```python
from build123d import *

# Parameters (mm, degrees)
F0_W           = 152.4
F0_H           = 134.62
F1_DEPTH       = 6.35
F3_D           = 3.9878
F3_CBORE_D     = 7.112
F3_CBORE_DEPTH = 4.000000001
F4_T1_DEPTH    = 124.46
F4_T3_DEPTH    = 142.24
F4_T5_DEPTH    = 13.97
F4_S9_W        = 5.08
F4_S9_H        = 5.08
F4_T10_DEPTH   = 5.08
F4_S15_W       = 5.08
F4_S15_H       = 5.08
F4_T16_DEPTH   = 5.08
F4_S21_W       = 5.08
F4_S21_H       = 5.08
F4_T22_DEPTH   = 5.08
F4_S27_W       = 5.08
F4_S27_H       = 5.08
F4_T28_DEPTH   = 5.08


# Not quite as in the source:
# - a fillet or chamfer that OpenCascade refuses, or shapes differently, is made with other operations: its cross-section is extruded or revolved along the edge and cut away or added
# - a feature names something its author has since deleted; it is built from what else it names


with BuildPart() as f1:
    # F0 (on Top) → F1 (new body)
    with BuildSketch(Plane.XY):
        Rectangle(F0_W, F0_H)
    extrude(amount=F1_DEPTH)

    # F3 (through all)
    with Locations(Plane.XY.offset(6.35)):
        with Locations((-72.39, 41.91), (-72.39, -34.29), (72.39, -34.29), (72.39, 41.91)):
            CounterBoreHole(F3_D / 2, F3_CBORE_D / 2, F3_CBORE_DEPTH)

    # F4: fillet of radius 5.08 on 8 edges, made by hand

    # F4_s2 → F4_t1 (cut)
    with BuildSketch(Plane.XZ.offset(-62.23)):
        with BuildLine():
            ThreePointArc((-76.2, 1.27), (-74.7121024484, 4.8621024484), (-71.12, 6.35))
            Line((-71.12, 6.35), (-76.2, 6.35))
            Line((-76.2, 6.35), (-76.2, 1.27))
        make_face()
        with BuildLine():
            ThreePointArc((76.2, 1.27), (74.7121024484, 4.8621024484), (71.12, 6.35))
            Line((71.12, 6.35), (76.2, 6.35))
            Line((76.2, 6.35), (76.2, 1.27))
        make_face()
    extrude(amount=F4_T1_DEPTH, mode=Mode.SUBTRACT)

    # F4_s4 → F4_t3 (cut)
    with BuildSketch(Plane.YZ.offset(-71.12)):
        with BuildLine():
            ThreePointArc((62.23, 6.35), (65.8221024484, 4.8621024484), (67.31, 1.27))
            Line((67.31, 1.27), (67.31, 6.35))
            Line((67.31, 6.35), (62.23, 6.35))
        make_face()
        with BuildLine():
            ThreePointArc((-67.31, 1.27), (-65.8221024484, 4.8621024484), (-62.23, 6.35))
            Line((-62.23, 6.35), (-67.31, 6.35))
            Line((-67.31, 6.35), (-67.31, 1.27))
        make_face()
    extrude(amount=F4_T3_DEPTH, mode=Mode.SUBTRACT)

    # F4_s6 → F4_t5 (cut)
    with BuildSketch(Plane.XY.offset(-12.7)):
        with BuildLine():
            ThreePointArc((-71.12, -67.31), (-74.7121024484, -65.8221024484), (-76.2, -62.23))
            Line((-76.2, -62.23), (-76.2, -67.31))
            Line((-76.2, -67.31), (-71.12, -67.31))
        make_face()
        with BuildLine():
            ThreePointArc((71.12, -67.31), (74.7121024484, -65.8221024484), (76.2, -62.23))
            Line((76.2, -62.23), (76.2, -67.31))
            Line((76.2, -67.31), (71.12, -67.31))
        make_face()
        with BuildLine():
            ThreePointArc((76.2, 62.23), (74.7121024484, 65.8221024484), (71.12, 67.31))
            Line((71.12, 67.31), (76.2, 67.31))
            Line((76.2, 67.31), (76.2, 62.23))
        make_face()
        with BuildLine():
            ThreePointArc((-76.2, 62.23), (-74.7121024484, 65.8221024484), (-71.12, 67.31))
            Line((-71.12, 67.31), (-76.2, 67.31))
            Line((-76.2, 67.31), (-76.2, 62.23))
        make_face()
    extrude(amount=F4_T5_DEPTH, mode=Mode.SUBTRACT)


with BuildPart() as f4_tool8:
    # F4_s9 → F4_t10 (new body)
    with BuildSketch(Plane.YZ.offset(-71.12)):
        with Locations((64.77, 3.81)):
            Rectangle(F4_S9_W, F4_S9_H)
    extrude(amount=-F4_T10_DEPTH)

    # F4_s11 → F4_t12 (revolve, cut)
    with BuildSketch(Plane(origin=(-71.12, 62.23, 1.27), x_dir=(0, -0.7071067812, -0.7071067812), z_dir=(0, 0.7071067812, -0.7071067812))):
        with BuildLine():
            ThreePointArc((0, -5.08), (5.08, 0), (0, 5.08))
            Line((0, 5.08), (0, -5.08))
        make_face()
    revolve(axis=Axis((-71.12, 62.23, 1.27), (-1, 0, 0)), mode=Mode.SUBTRACT)


with BuildPart() as f1_1:
    add(f1.part)

    # F4_t7: cut F4_tool8
    add(f4_tool8.part, mode=Mode.SUBTRACT)


with BuildPart() as f4_tool14:
    # F4_s15 → F4_t16 (new body)
    with BuildSketch(Plane.XZ.offset(62.23)):
        with Locations((-73.66, 3.81)):
            Rectangle(F4_S15_W, F4_S15_H)
    extrude(amount=F4_T16_DEPTH)

    # F4_s17 → F4_t18 (revolve, cut)
    with BuildSketch(Plane(origin=(-71.12, -62.23, 1.27), x_dir=(0.7071067812, 0, -0.7071067812), z_dir=(-0.7071067812, 0, -0.7071067812))):
        with BuildLine():
            ThreePointArc((0, -5.08), (5.08, 0), (0, 5.08))
            Line((0, 5.08), (0, -5.08))
        make_face()
    revolve(axis=Axis((-71.12, -62.23, 1.27), (0, -1, 0)), mode=Mode.SUBTRACT)


with BuildPart() as f1_2:
    add(f1_1.part)

    # F4_t13: cut F4_tool14
    add(f4_tool14.part, mode=Mode.SUBTRACT)


with BuildPart() as f4_tool20:
    # F4_s21 → F4_t22 (new body)
    with BuildSketch(Plane.YZ.offset(71.12)):
        with Locations((64.77, 3.81)):
            Rectangle(F4_S21_W, F4_S21_H)
    extrude(amount=F4_T22_DEPTH)

    # F4_s23 → F4_t24 (revolve, cut)
    with BuildSketch(Plane(origin=(71.12, 62.23, 1.27), x_dir=(0, -0.7071067812, -0.7071067812), z_dir=(0, -0.7071067812, 0.7071067812))):
        with BuildLine():
            ThreePointArc((0, -5.08), (5.08, 0), (0, 5.08))
            Line((0, 5.08), (0, -5.08))
        make_face()
    revolve(axis=Axis((71.12, 62.23, 1.27), (1, 0, 0)), mode=Mode.SUBTRACT)


with BuildPart() as f1_3:
    add(f1_2.part)

    # F4_t19: cut F4_tool20
    add(f4_tool20.part, mode=Mode.SUBTRACT)


with BuildPart() as f4_tool26:
    # F4_s27 → F4_t28 (new body)
    with BuildSketch(Plane.XZ.offset(62.23)):
        with Locations((73.66, 3.81)):
            Rectangle(F4_S27_W, F4_S27_H)
    extrude(amount=F4_T28_DEPTH)

    # F4_s29 → F4_t30 (revolve, cut)
    with BuildSketch(Plane(origin=(71.12, -62.23, 1.27), x_dir=(-0.7071067812, 0, -0.7071067812), z_dir=(-0.7071067812, 0, 0.7071067812))):
        with BuildLine():
            ThreePointArc((0, -5.08), (5.08, 0), (0, 5.08))
            Line((0, 5.08), (0, -5.08))
        make_face()
    revolve(axis=Axis((71.12, -62.23, 1.27), (0, -1, 0)), mode=Mode.SUBTRACT)


with BuildPart() as f1_4:
    add(f1_3.part)

    # F4_t25: cut F4_tool26
    add(f4_tool26.part, mode=Mode.SUBTRACT)


solid = f1_4.part
```
Input: part model. Units: mm. Frame: model coordinates. A direction names the side the tool comes from. Coordinates: 2 decimals unless noted, no trailing zeros. Loops run counter-clockwise (first coordinate to the right, second up) from the corner with the lowest first, then second, coordinate; pieces in that order, holes last. Notation, with made-up numbers: M 57,6.25 L 83,6.25 A27 cw 83,31.25 Z; hole C 18,-40 d7. An arc over 180 degrees is marked long. Use a Markdown table: item, result. Add a question column.
1) Set-up query: faces 1 (the cylindrical face through (-70.808, 40.697, 1.159)), 2 (the flat face through (74, -36, 2.35)). Return all of +Z, -Z, +X, -X, +Y, -Y with unobstructed straight access to the full face (end or side cutting, diameter ignored); none if empty.
2) Draft query along X for faces 3 (the cylindrical face through (74.751, 65.782, 0.626)), 4 (the flat face through (-1, 1, 0)), 5 (the flat face through (-71, 40, 2.35)). Return one class per face: +X half, -X half, draft (parallel to the pull), parting line (faces both ways), or undercut.
3) Section A-A, the plane y = -34.29. Return the cut outline in (x, z).
4) Line query: L1, parallel to Y at x = 72.39, z = 0.9; L2, parallel to X at y = -34.29, z = 5.2; L3, parallel to X at y = -1.5, z = 1.75. Output: solid intervals per line, ascending. Write a range as from..to.
5) Pin query (flat end, axial travel): P1, Ø3, axis at y = 2, z = 4, coming from the +X side; P2, Ø2.5, axis at x = -72.39, y = 41.91, coming from the +Z side; P3, Ø2, axis at x = -71, y = 43, coming from the +Z side; P4, Ø2, axis at y = 33, z = 5.5, coming from the +X side. Return the tip coordinate at first contact, or that it passes through.
6) Section B-B, the plane z = 4.5. Return the cut outline in (x, y).
Answer below:
| question | item | result |
|---|---|---|
| 1 | face 1 | +Z, -Z |
| 1 | face 2 | +Z |
| 2 | face 3 | +X half |
| 2 | face 4 | draft |
| 2 | face 5 | undercut |
| 3 | outline | M -76.2,0 L -74.38,0 L -74.38,2.35 L -75.95,2.35 L -75.95,2.86 A5.08 ccw -76.2,1.27 Z; M -70.4,0 L 70.4,0 L 70.4,2.35 L 68.83,2.35 L 68.83,6.35 L -68.83,6.35 L -68.83,2.35 L -70.4,2.35 Z; M 74.38,0 L 76.2,0 L 76.2,1.27 A5.08 ccw 75.95,2.86 L 75.95,2.35 L 74.38,2.35 Z |
| 4 | L1 | -67.15..-36.28, -32.3..39.92, 43.9..67.15 |
| 4 | L2 | -68.83..68.83 |
| 4 | L3 | -76.18..76.18 |
| 5 | P1 | x = 76.05 |
| 5 | P2 | through |
| 5 | P3 | z = 2.35 |
| 5 | P4 | x = 75.04 |
| 6 | outline | M -75.04,-62.23 A3.92 ccw -71.12,-66.15 L 71.12,-66.15 A3.92 ccw 75.04,-62.23 L 75.04,-36.66 A3.56 cw long 75.04,-31.92 L 75.04,39.54 A3.56 cw long 75.04,44.28 L 75.04,62.23 A3.92 ccw 71.12,66.15 L -71.12,66.15 A3.92 ccw -75.04,62.23 L -75.04,44.28 A3.56 cw long -75.04,39.54 L -75.04,-31.92 A3.56 cw long -75.04,-36.66 Z |
